from build123d import *

# Parameters (mm, degrees)
EXTRUDE_START                      = 0.1
EXTRUDE_726_DEPTH                  = 2.9
EXTRUDE_1021_DEPTH                 = 0.1
EXTRUDE_1021_DEPTH_BACK            = 1
SKETCH_2_R                         = 2.85
FILLET_1_R                         = 0.05
EXTRUDE_START_2                    = -0.3
EXTRUDE_1608_DEPTH                 = 1
CUT_EXTRUDE_8_DEPTH                = 0.2
EXTRUDE_START_3                    = 0.05
SKETCH_9_R                         = 0.046
EXTRUDE_1_DEPTH                    = 0.461
EXTRUDE_1_OTHER_WAY_DEPTH          = 0.05
EXTRUDE_1_OTHER_WAY_DRAFT          = 45
PATTERN_CIRCULAR_3_COUNT           = 2
PATTERN_START                      = 0.05
PATTERN_CIRCULAR_3_COPY_1_SKETCH_R = 0.046
PATTERN_CIRCULAR_3_COPY_1_DEPTH    = 0.05
PATTERN_CIRCULAR_3_COPY_1_DRAFT    = 45
PATTERN_CIRCULAR_3_COPY_2_SKETCH_R = 0.046
PATTERN_CIRCULAR_3_COPY_2_DEPTH    = 0.05
PATTERN_CIRCULAR_3_COPY_2_DRAFT    = 45
EXTRUDE_4261_DEPTH                 = 0.1


with BuildPart() as part:
    # Эскиз1 → Extrude 726 (new body)
    with BuildSketch(Plane.XY.offset(EXTRUDE_START)):
        with BuildLine():
            Line((-2.85, -1.75), (-1.75, -2.85))
            Line((-1.75, -2.85), (2.35, -2.85))
            ThreePointArc((2.35, -2.85), (2.703553391, -2.703553391), (2.85, -2.35))
            Line((2.85, -2.35), (2.85, 1.75))
            Line((2.85, 1.75), (1.75, 2.85))
            Line((1.75, 2.85), (-2.35, 2.85))
            ThreePointArc((-2.35, 2.85), (-2.703553391, 2.703553391), (-2.85, 2.35))
            Line((-2.85, 2.35), (-2.85, -1.75))
        make_face()
    extrude(amount=EXTRUDE_726_DEPTH)

    # Эскиз2 → Extrude 1021 (add, two sides: drawn at the far end of the back side and taken through both)
    with BuildSketch(Plane.XY.offset(3).offset(-EXTRUDE_1021_DEPTH_BACK)):
        Circle(SKETCH_2_R)
    extrude(amount=EXTRUDE_1021_DEPTH + EXTRUDE_1021_DEPTH_BACK)

    # Скругление1
    fillet_1_edges = [part.edges().sort_by_distance(p)[0] for p in [
        (-2.85, 0, 3.1),
    ]]
    fillet(fillet_1_edges, radius=FILLET_1_R)

    # Эскиз6 → Extrude 1608 (add)
    with BuildSketch(Plane(origin=(0.55, -0.55, 0), x_dir=(0, 0, 1), z_dir=(0.7071067811865498, -0.7071067811865452, 0)).offset(EXTRUDE_START_2)):
        with BuildLine():
            Line((2.908, -3.347691193), (2.995, -3.295691193))
            Line((2.995, -3.295691193), (2.995, -3.265691193))
            Line((2.995, -3.265691193), (0.125, -3.265691193))
            Line((0.125, -3.265691193), (0.125, -2.765691193))
            Line((0.125, -2.765691193), (0, -2.765691193))
            Line((0, -2.765691193), (0, -3.295691193))
            Line((0, -3.295691193), (2.715, -3.295691193))
            add(Edge.make_bspline(
                [(2.715, -3.295691193), (2.818817166, -3.299465526), (2.908, -3.347691193)],
                knots=[0, 0, 0, 1, 1, 1], degree=2))
        make_face()
    extrude_1608 = extrude(amount=-EXTRUDE_1608_DEPTH)

    # Эскиз8 → Вытянуть8 (cut)
    with BuildSketch(Plane.XY.offset(3)):
        Polygon((2.512132034, 2.087867966), (2.087867966, 2.512132034), (1.735728789, 2.159992857), (2.159992857, 1.735728789), align=None)
        Polygon((-1.687867966, -2.112132034), (-1.342499119, -1.753350263), (-1.774766314, -1.337243218), (-2.12013516, -1.69602499), align=None)
    extrude(amount=-CUT_EXTRUDE_8_DEPTH, mode=Mode.SUBTRACT)

    # Эскиз9 → Бобышка-Вытянуть1 (add)
    with BuildSketch(Plane(origin=(2.309192388, 2.309192388, 0), x_dir=(0, 0, 1), z_dir=(-0.7071067811865452, -0.7071067811865498, 0)).offset(EXTRUDE_START_3)):
        with Locations(Location((2.899, 0, 0), (0, 0, 270))):
            Circle(SKETCH_9_R)
    extrude_1 = extrude(amount=EXTRUDE_1_DEPTH)


with BuildPart() as extrude_1_other_way_tool:
    # Эскиз9 → Бобышка-Вытянуть1 other way (with draft: the straight prism first)
    with BuildSketch(Plane(origin=(2.309192388, 2.309192388, 0), x_dir=(0, 0, 1), z_dir=(-0.7071067811865452, -0.7071067811865498, 0)).offset(EXTRUDE_START_3)):
        with Locations(Location((2.899, 0, 0), (0, 0, 270))):
            Circle(SKETCH_9_R)
    extrude(amount=-EXTRUDE_1_OTHER_WAY_DEPTH)
    # Бобышка-Вытянуть1 other way: the draft: its side faces are tilted about the plane it starts from
    extrude_1_other_way_sides = [extrude_1_other_way_tool.faces().sort_by_distance(p)[0] for p in [
        (2.258987807, 2.324041631, 2.899),
    ]]
    draft(extrude_1_other_way_sides, Plane(origin=(2.309192388, 2.309192388, 0), x_dir=(0, 0, 1), z_dir=(-0.7071067811865452, -0.7071067811865498, 0)).offset(EXTRUDE_START_3), EXTRUDE_1_OTHER_WAY_DRAFT)


with BuildPart() as part_1:
    add(part.part)

    # Бобышка-Вытянуть1 other way: add extrude_1_other_way_tool
    add(extrude_1_other_way_tool.part)

    # Круговой массив3: Extrude 1608, Бобышка-Вытянуть1 ×2 about axis
    pattern_circular_3_axis = Axis((0, 0, 3.1), (0, 0, -1))
    add([extrude_1608.rotate(pattern_circular_3_axis, i * 360 / PATTERN_CIRCULAR_3_COUNT) for i in range(1, PATTERN_CIRCULAR_3_COUNT)])
    add([extrude_1.rotate(pattern_circular_3_axis, i * 360 / PATTERN_CIRCULAR_3_COUNT) for i in range(1, PATTERN_CIRCULAR_3_COUNT)])


with BuildPart() as pattern_circular_3_copy_1_tool:
    # Круговой массив3 copy 1 sketch → Круговой массив3 copy 1 (with draft: the straight prism first)
    with BuildSketch(Plane(origin=(-2.309192388, -2.309192388, 0), x_dir=(0, 0, 1), z_dir=(0.7071067811865451, 0.7071067811865499, 0)).offset(PATTERN_START)):
        with Locations(Location((2.899, 0, 0), (0, 0, 270))):
            Circle(PATTERN_CIRCULAR_3_COPY_1_SKETCH_R)
    extrude(amount=-PATTERN_CIRCULAR_3_COPY_1_DEPTH)
    # Круговой массив3 copy 1: the draft: its side faces are tilted about the plane it starts from
    pattern_circular_3_copy_1_sides = [pattern_circular_3_copy_1_tool.faces().sort_by_distance(p)[0] for p in [
        (-2.258987807, -2.324041631, 2.899),
    ]]
    draft(pattern_circular_3_copy_1_sides, Plane(origin=(-2.309192388, -2.309192388, 0), x_dir=(0, 0, 1), z_dir=(0.7071067811865451, 0.7071067811865499, 0)).offset(PATTERN_START), PATTERN_CIRCULAR_3_COPY_1_DRAFT)


with BuildPart() as part_2:
    add(part_1.part)

    # Круговой массив3 copy 1: add pattern_circular_3_copy_1_tool
    add(pattern_circular_3_copy_1_tool.part)


with BuildPart() as pattern_circular_3_copy_2_tool:
    # Круговой массив3 copy 2 sketch → Круговой массив3 copy 2 (with draft: the straight prism first)
    with BuildSketch(Plane(origin=(-2.309192388, -2.309192388, 0), x_dir=(0, 0, 1), z_dir=(0.7071067811865451, 0.7071067811865499, 0)).offset(PATTERN_START)):
        with Locations(Location((2.899, 0, 0), (0, 0, 270))):
            Circle(PATTERN_CIRCULAR_3_COPY_2_SKETCH_R)
    extrude(amount=-PATTERN_CIRCULAR_3_COPY_2_DEPTH)
    # Круговой массив3 copy 2: the draft: its side faces are tilted about the plane it starts from
    pattern_circular_3_copy_2_sides = [pattern_circular_3_copy_2_tool.faces().sort_by_distance(p)[0] for p in [
        (-2.258987807, -2.324041631, 2.899),
    ]]
    draft(pattern_circular_3_copy_2_sides, Plane(origin=(-2.309192388, -2.309192388, 0), x_dir=(0, 0, 1), z_dir=(0.7071067811865451, 0.7071067811865499, 0)).offset(PATTERN_START), PATTERN_CIRCULAR_3_COPY_2_DRAFT)


with BuildPart() as part_3:
    add(part_2.part)

    # Круговой массив3 copy 2: add pattern_circular_3_copy_2_tool
    add(pattern_circular_3_copy_2_tool.part)

    # Эскиз13 → Extrude 4261 (add)
    with BuildSketch(Plane(origin=(0, 0, 0.1), x_dir=(-1, 0, 0), z_dir=(0, 0, -1))):
        with BuildLine():
            Line((2.050035735, 1.148848765), (2.8, 1.148848765))
            Line((2.8, 1.148848765), (2.8, 1.728848765))
            Line((2.8, 1.728848765), (1.728848765, 2.8))
            Line((1.728848765, 2.8), (-1.728848765, 2.8))
            Line((-1.728848765, 2.8), (-2.8, 1.728848765))
            Line((-2.8, 1.728848765), (-2.8, 1.148848765))
            Line((-2.8, 1.148848765), (-2.050035735, 1.148848765))
            ThreePointArc((-2.050035735, 1.148848765), (0, 2.35), (2.050035735, 1.148848765))
        make_face()
        with BuildLine():
            Line((-2.8, -1.148848765), (-2.050035735, -1.148848765))
            ThreePointArc((-2.050035735, -1.148848765), (0, -2.35), (2.050035735, -1.148848765))
            Line((2.050035735, -1.148848765), (2.8, -1.148848765))
            Line((2.8, -1.148848765), (2.8, -1.728848765))
            Line((2.8, -1.728848765), (1.728848765, -2.8))
            Line((1.728848765, -2.8), (-1.728848765, -2.8))
            Line((-1.728848765, -2.8), (-2.8, -1.728848765))
            Line((-2.8, -1.728848765), (-2.8, -1.148848765))
        make_face()
    extrude(amount=EXTRUDE_4261_DEPTH)


solid = part_3.part
Model file for the job. Use its own axes, mm. A direction names the side the tool comes from. Coordinates: 2 decimals unless noted, no trailing zeros. Return JSON: item names as keys, results as strings. Group by question number.
Item 1: Tool access for faces 5 (the flat face through (2.2, -2.2, 3)), 6 (the flat face through (-2.2, 2.3, 3)), 7 (the flat face through (2.85, 0, 2)), 8 (the flat face through (-2.2, -2.1, 3)), 9 (the flat face through (0.04, 2.54, 0)): list every direction of +Z, -Z, +X, -X, +Y, -Y with a clear straight run to the whole face (end or side of a thin tool).
Item 2: Pull direction Y, two halves, no side cores. Call faces 1 (the flat face through (0, 2.85, 2)), 2 (the flat face through (0, 0, 0.1)), 3 (the flat face through (0, -2.85, 2)), 4 (the flat face through (-2.85, 0, 2)): pulls with the +Y half, pulls with the -Y half, needs draft (parallel to the pull), parting line crosses it, or undercut.
Item 3: Flat gauge pin, fed straight in: P1, Ø1, axis at x = 0, y = 0.5, coming from the -Z side. Where does the tip first touch, or does it go through?
Item 4: Wall check: line 1 along Z through (x, y) = (2.65, -1.45); line 2 along Z through (x, y) = (1.55, 0.95); line 3 along X through (y, z) = (1.9, 0.9). Give the ranges that are in metal, low to high. Write a range as [from, to].
Item 5: Saw through at A-A on z = 0.55. State how many separate pieces and enclosed holes the cut face has, then the cut area to 3 significant figures.
Values found:
{
 "1": {"face 5": "+Z, +X, -Y", "face 6": "+Z, -X, +Y", "face 7": "+Z, -Z, +X, +Y, -Y", "face 8": "+Z, -X, -Y", "face 9": "-Z, +X, -X, +Y, -Y"},
 "2": {"face 1": "pulls with the +Y half", "face 2": "undercut", "face 3": "pulls with the -Y half", "face 4": "needs draft"},
 "3": {"P1": "stops at z = 0.1"},
 "4": {"line 1": "z = [0, 3]", "line 2": "z = [0.1, 3.1]", "line 3": "x = [-2.85, 2.7]"},
 "5": {"separate pieces": "3", "enclosed holes": "0", "area": "31.2 mm2"}
}
